from build123d import *

# Parameters (mm, degrees)
F0_R         = 2.75
F1_DEPTH     = 38
F3_DEPTH     = 3
F5_DEPTH     = 25
F6_SIZE2     = 5
F6_SIZE      = 8
F7_SIZE2     = 6.5
F7_SIZE      = 15
F8_SIZE2     = 6
F8_SIZE      = 10
F9_SIZE2     = 10
F9_SIZE      = 6
F10_R        = 2
F11_C1_SIZE2 = 10
F11_C1_SIZE  = 5.5
F11_C2_SIZE2 = 10
F11_C2_SIZE  = 5.5
F12_SIZE2    = 5.5
F12_SIZE     = 10
F12_2_SIZE2  = 5.5
F12_2_SIZE   = 10
F13_R        = 5
F14_R        = 5
F15_T1_DEPTH = 34.34956364
F15_T3_DEPTH = 11.5008904579
F15_T6_ANGLE = 180


# Not quite as in the source:
# - a fillet or chamfer that OpenCascade refuses, or shapes differently, is made with other operations: its cross-section is extruded or revolved along the edge and cut away or added


with BuildPart() as f1:
    # F0 (on Top) → F1 (new body)
    with BuildSketch(Plane.XY):
        with BuildLine():
            Line((-17, 25), (-20, 25))
            Line((-20, 25), (-20, 0))
            Line((-20, 0), (20, 0))
            Line((20, 0), (20, 25))
            Line((20, 25), (17, 25))
            Line((17, 25), (17, 19.1485292704))
            ThreePointArc((17, 19.1485292704), (16.286002286, 17.205800893), (14.4838709677, 16.1878082625))
            ThreePointArc((14.4838709677, 16.1878082625), (12.7404153064, 15.5329250756), (11.3827554868, 14.2580645161))
            ThreePointArc((11.3827554868, 14.2580645161), (10.3140016776, 13.332997333), (8.9402852679, 13))
            Line((8.9402852679, 13), (-8.9402852679, 13))
            ThreePointArc((-8.9402852679, 13), (-10.3140016776, 13.332997333), (-11.3827554868, 14.2580645161))
            ThreePointArc((-11.3827554868, 14.2580645161), (-12.7404153064, 15.5329250756), (-14.4838709677, 16.1878082625))
            ThreePointArc((-14.4838709677, 16.1878082625), (-16.286002286, 17.205800893), (-17, 19.1485292704))
            Line((-17, 19.1485292704), (-17, 25))
        make_face()
        with Locations((-15.25, 11.5)):
            Circle(F0_R, mode=Mode.SUBTRACT)
        with Locations((15.25, 11.5)):
            Circle(F0_R, mode=Mode.SUBTRACT)
    extrude(amount=F1_DEPTH)

    # F2 (on face) → F3 (cut)
    with BuildSketch(Plane(origin=(0, 0, 0), x_dir=(1, 0, 0), z_dir=(0, 0, -1))):
        with BuildLine():
            Line((18, -7.8), (-18, -7.8))
            ThreePointArc((-18, -7.8), (-19.4142135624, -8.3857864376), (-20, -9.8))
            Line((-20, -9.8), (-20, -60))
            Line((-20, -60), (20, -60))
            Line((20, -60), (20, -9.8))
            ThreePointArc((20, -9.8), (19.4142135624, -8.3857864376), (18, -7.8))
        make_face()
    extrude(amount=-F3_DEPTH, mode=Mode.SUBTRACT)

    # F4 (on face) → F5 (cut)
    with BuildSketch(Plane.XZ):
        with BuildLine():
            Line((-9.25, 38), (-9.25, 20.5))
            ThreePointArc((-9.25, 20.5), (0, 11.25), (9.25, 20.5))
            Line((9.25, 20.5), (9.25, 38))
            Line((9.25, 38), (-9.25, 38))
        make_face()
    extrude(amount=-F5_DEPTH, mode=Mode.SUBTRACT)

    # F6
    f6_edges = [f1.edges().sort_by_distance(p)[0] for p in [
        (0, 0, 0),
    ]]
    f6_side = f1.faces().sort_by_distance((0, 0, 0.551725))[0]
    chamfer(f6_edges, length=F6_SIZE, length2=F6_SIZE2, reference=f6_side)

    # F7
    f7_edges = [f1.edges().sort_by_distance(p)[0] for p in [
        (-14.625, 0, 38),
        (14.625, 0, 38),
    ]]
    f7_side = f1.faces().sort_by_distance((19.5, 0, 23))[0]
    chamfer(f7_edges, length=F7_SIZE, length2=F7_SIZE2, reference=f7_side)

    # F8
    f8_edges = [f1.edges().sort_by_distance(p)[0] for p in [
        (20, 0, 15.5),
    ]]
    f8_side = f1.faces().sort_by_distance((20, 13.094719, 19.529129))[0]
    chamfer(f8_edges, length=F8_SIZE, length2=F8_SIZE2, reference=f8_side)

    # F9
    f9_edges = [f1.edges().sort_by_distance(p)[0] for p in [
        (-20, 0, 15.5),
    ]]
    f9_side = f1.faces().sort_by_distance((11.625, 0, 22.628382))[0]
    chamfer(f9_edges, length=F9_SIZE, length2=F9_SIZE2, reference=f9_side)

    # F10
    f10_edges = [f1.edges().sort_by_distance(p)[0] for p in [
        (15.95, 3.25, 30.5),
        (-15.95, 3.25, 30.5),
        (14, 0, 15.5),
        (-14, 0, 15.5),
        (-15.5, 2.5, 4),
        (15.5, 2.5, 4),
    ]]
    fillet(f10_edges, radius=F10_R)

    # F11: chamfer of 10 x 5.5 on 2 edges, made by hand

    # F11_c1
    f11_c1_edges = [f1.edges().sort_by_distance(p)[0] for p in [
        (-18.5, 25, 3),
    ]]
    f11_c1_side = f1.faces().sort_by_distance((-18.5, 24.89, 3))[0]
    chamfer(f11_c1_edges, length=F11_C1_SIZE, length2=F11_C1_SIZE2, reference=f11_c1_side)

    # F11_c2
    f11_c2_edges = [f1.edges().sort_by_distance(p)[0] for p in [
        (18.5, 25, 3),
    ]]
    f11_c2_side = f1.faces().sort_by_distance((18.5, 24.89, 3))[0]
    chamfer(f11_c2_edges, length=F11_C2_SIZE, length2=F11_C2_SIZE2, reference=f11_c2_side)

    # F12
    f12_edges = [f1.edges().sort_by_distance(p)[0] for p in [
        (18.5, 25, 38),
    ]]
    f12_side = f1.faces().sort_by_distance((18.5, 25, 25.5))[0]
    chamfer(f12_edges, length=F12_SIZE, length2=F12_SIZE2, reference=f12_side)

    # F12#2
    f12_2_edges = [f1.edges().sort_by_distance(p)[0] for p in [
        (-18.5, 25, 38),
    ]]
    f12_2_side = f1.faces().sort_by_distance((-18.5, 25, 25.5))[0]
    chamfer(f12_2_edges, length=F12_2_SIZE, length2=F12_2_SIZE2, reference=f12_2_side)

    # F13
    f13_edges = [f1.edges().sort_by_distance(p)[0] for p in [
        (20, 10, 20.5),
        (-20, 10, 20.5),
    ]]
    fillet(f13_edges, radius=F13_R)

    # F14
    f14_edges = [f1.edges().sort_by_distance(p)[0] for p in [
        (18.5, 25, 28),
        (18.5, 25, 13),
        (-18.5, 25, 13),
        (-18.5, 25, 28),
    ]]
    fillet(f14_edges, radius=F14_R)

    # F15: chamfer of 3.5 on 5 edges, made by hand

    # F15_s2 → F15_t1 (cut)
    with BuildSketch(Plane(origin=(0, 4.8121986531, 11.1050738149), x_dir=(1, 0, 0), z_dir=(0, 0.3976074376, 0.9175556253))):
        Polygon((-12.75, -9.1449710656), (-9.25, -5.6449710656), (-9.25, -9.1449710656), align=None)
        Polygon((9.25, -5.6449710656), (12.75, -9.1449710656), (9.25, -9.1449710656), align=None)
    extrude(amount=F15_T1_DEPTH, mode=Mode.SUBTRACT)

    # F15_s4 → F15_t3 (cut)
    with BuildSketch(Plane.XY.offset(20.5)):
        Polygon((-9.25, 3.5), (-12.75, 0), (-9.25, 0), align=None)
        Polygon((12.75, 0), (9.25, 3.5), (9.25, 0), align=None)
    extrude(amount=F15_T3_DEPTH, mode=Mode.SUBTRACT)

    # F15_s5 → F15_t6 (revolve, cut)
    with BuildSketch(Plane.XY.offset(20.5)):
        Polygon((-12.75, 0), (-9.25, 3.5), (-9.25, 0), align=None)
    revolve(axis=Axis((0, 0, 20.5), (0, -1, 0)), revolution_arc=F15_T6_ANGLE, mode=Mode.SUBTRACT)


solid = f1.part
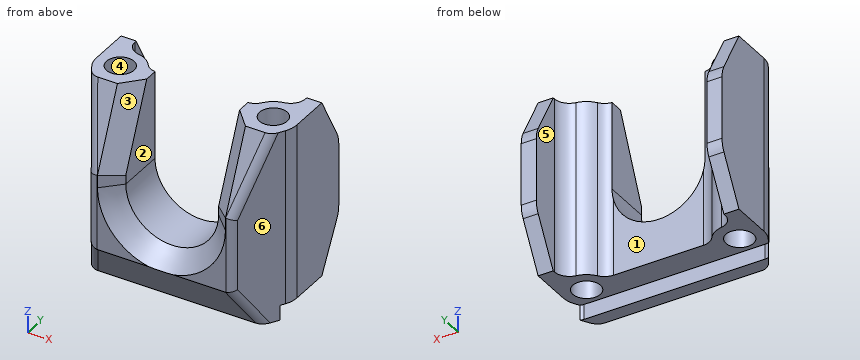
Build history of the part. All positions in model axes, mm. Face numbers are marked on the shaded views. A direction names the side the tool comes from. Round coordinates to 2 decimals unless told otherwise and drop trailing zeros. Order: outer loops, then holes, each group sorted by start corner. A loop starts at its lowest first (then second) coordinate and runs counter-clockwise, first axis right, second up. Notation, with made-up numbers: M 4,78.5 L 11,78.5 A15 cw 11,83.5 Z; hole C 35.5,12 d1. An arc over 180 degrees is marked long. Use CSV: the item, a comma, the result in double quotes. Start each with the question number.
(1) Mould opens along Y. For the marked faces 4, 5 and 6 say: +Y half, -Y half, draft (parallel to the pull), parting line (faces both ways), or undercut.
(2) Tool access for the marked faces 1, 2 and 3: list every direction of +Z, -Z, +X, -X, +Y, -Y with a clear straight run to the whole face (end or side of a thin tool).
(3) Cut at D-D on y = 15. List the corners of the cut face in (x, z).
(4) Drill centre lines: probe 1 along X at (y, z) = (11.5, 24); probe 2 along X at (y, z) = (11.5, 13.5); probe 3 along X at (y, z) = (19, 8). Where is each one in solid material? Low to high.
(5) Cut at C-C on x = 0. List the corners of the cut face in (y, z).
(6) Cut at A-A on y = 20.75. List the corners of the cut face in (x, z).
(7) Cut at B-B on z = 24.5. State how many separate pieces and enclosed holes the cut face has, then the cut area to 3 significant figures.
(8) Flat gauge pins, fed straight in: P1, Ø5, axis at x = -7, z = 19.5, coming from the +Y side; P2, Ø2, axis at x = -5.5, z = 16.5, coming from the -Y side; P3, Ø12, axis at x = -2, z = 11.5, coming from the +Y side; P4, Ø8, axis at x = 4.5, y = 15.5, coming from the -Z side. Where does each tip first touch, or does it go through?
Findings:
1,face 4,"undercut"
1,face 5,"draft"
1,face 6,"-Y half"
2,face 1,"+Z, -Z, +Y"
2,face 2,"+Z, +Y, -Y"
2,face 3,"+Z, -Y"
3,outline,"M -20,3 L -12.04,3 L -12.04,38 L -20,38 Z; M 12.04,3 L 20,3 L 20,38 L 12.04,38 Z"
4,probe 1,"x = -20 to -18, -12.5 to -9.25, 9.25 to 12.5, 18 to 20"
4,probe 2,"x = -20 to -18, -12.5 to -6.05, 6.05 to 12.5, 18 to 20"
4,probe 3,"x = -20 to -17, 17 to 20"
5,outline,"M 0.1,7.85 L 5,0 L 7.8,0 L 7.8,3 L 13,3 L 13,11.25 L 3.5,11.25 Z"
6,outline,"M -20,5.27 L -17,5.27 L -17,35.73 L -20,35.73 Z; M 17,5.27 L 20,5.27 L 20,35.73 L 17,35.73 Z"
7,separate pieces,"2"
7,enclosed holes,"2"
7,area,"260 mm^2"
8,P1,"stops at y = 13.05"
8,P2,"passes through"
8,P3,"stops at y = 13"
8,P4,"stops at z = 3"
